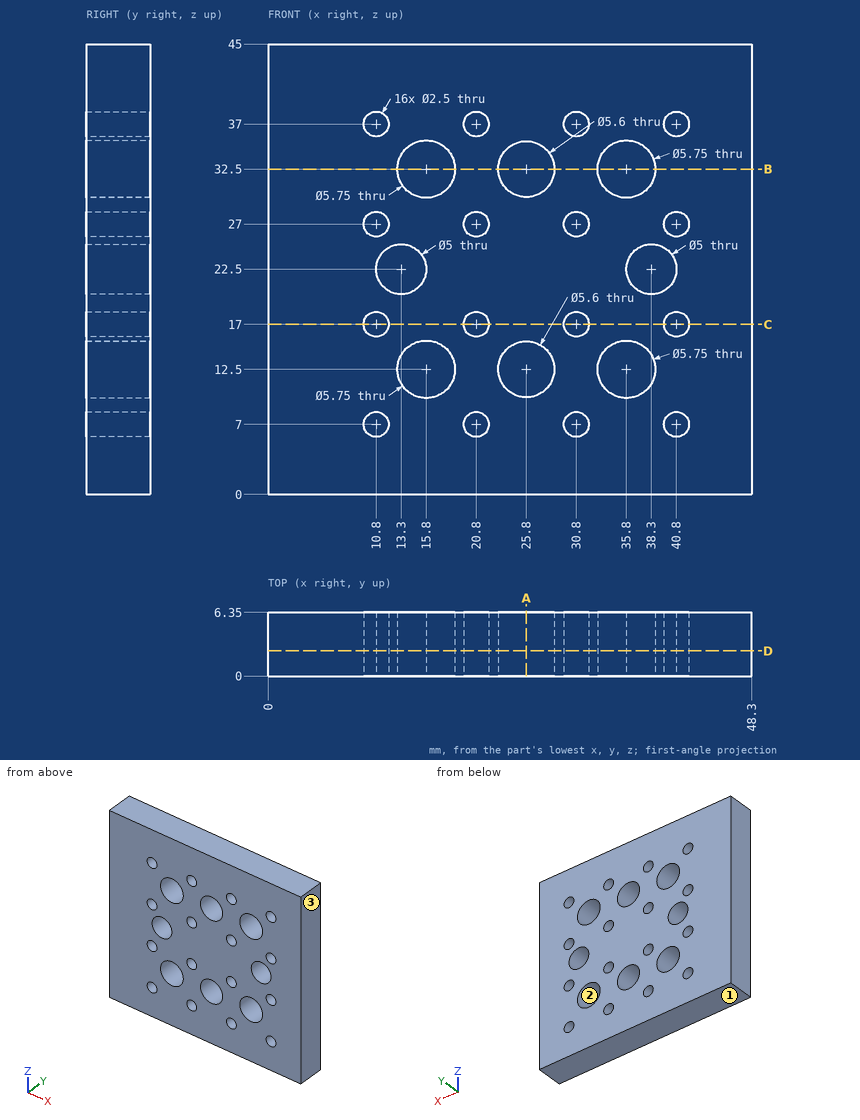
Input: dimensioned drawing with shaded views. Units: mm. Origin: part minimum x, y, z. Give positions to 0.01 mm unless a question says otherwise; leave off trailing zeros. Order: outer loops, then holes, each group sorted by start corner. A loop starts at its lowest first (then second) coordinate and runs counter-clockwise, first axis right, second up. Notation, with made-up numbers: (51, 12.5) -> (74, 12.5) arc R11 cw to (74, 33.5) -> close; hole circle Ø4 at (34, 46.5). An arc over 180 degrees is marked (long way). Write item = value, one per line.
Item 1: Section query D-D (y = 2.5). State how many separate pieces and enclosed holes the cut face has, then the cut area to 3 significant figures.
Check result:
separate_pieces = 1
enclosed_holes = 24
area = 1,900 mm²
Item 2: Section query C-C (z = 17). Output: boundary loops of the cut face in (x, y).
Check result:
outline = (0, 0) -> (9.55, 0) -> (9.55, 6.35) -> (0, 6.35) -> close; (12.05, 0) -> (19.55, 0) -> (19.55, 6.35) -> (12.05, 6.35) -> close; (22.05, 0) -> (29.55, 0) -> (29.55, 6.35) -> (22.05, 6.35) -> close; (32.05, 0) -> (39.55, 0) -> (39.55, 6.35) -> (32.05, 6.35) -> close; (42.05, 0) -> (48.3, 0) -> (48.3, 6.35) -> (42.05, 6.35) -> close
Item 3: Section query A-A (x = 25.8). Output: boundary loops of the cut face in (y, z), then the cut area to 3 significant figures.
Check result:
outline = (0, 0) -> (6.35, 0) -> (6.35, 9.7) -> (0, 9.7) -> close; (0, 15.3) -> (6.35, 15.3) -> (6.35, 29.7) -> (0, 29.7) -> close; (0, 35.3) -> (6.35, 35.3) -> (6.35, 45) -> (0, 45) -> close
area = 215 mm²
Item 4: Mould query, pull axis X, two halves, no side actions, for the marked faces 1, 2 and 3. Classes: +X half, -X half, draft (parallel to the pull), parting line (faces both ways), or undercut.
Check result:
face_1 = draft
face_2 = undercut
face_3 = +X half
Item 5: Contact query for a flat-ended pin moving along its axis: pin 1 (3 mm diameter, centred on x = 20.8, z = 27, fed in from +Y). Output: stop coordinate, or through.
Check result:
pin_1 = 6.35
Item 6: Section query B-B (z = 32.5). Output: boundary loops of the cut face in (x, y) (3 decimals).
Check result:
outline = (0, 0) -> (12.925, 0) -> (12.925, 6.35) -> (0, 6.35) -> close; (18.675, 0) -> (23, 0) -> (23, 6.35) -> (18.675, 6.35) -> close; (28.6, 0) -> (32.925, 0) -> (32.925, 6.35) -> (28.6, 6.35) -> close; (38.675, 0) -> (48.3, 0) -> (48.3, 6.35) -> (38.675, 6.35) -> close
Item 7: Ray query, probe 1 along X at (y, z) = (1.5, 32.5) (3 decimals); probe 2 along X at (y, z) = (3.5, 37); probe 3 along X at (y, z) = (0.75, 23). Return the intervals inside material, ascending.
Check result:
probe_1 = 0 to 12.925, 18.675 to 23, 28.6 to 32.925, 38.675 to 48.3
probe_2 = 0 to 9.55, 12.05 to 19.55, 22.05 to 29.55, 32.05 to 39.55, 42.05 to 48.3
probe_3 = 0 to 10.85, 15.75 to 35.85, 40.75 to 48.3
